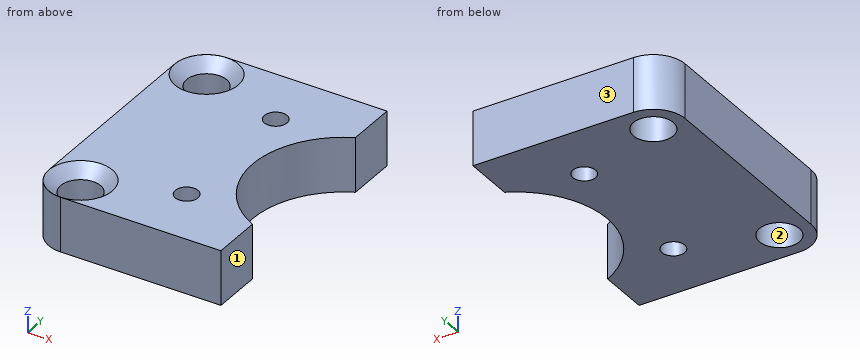
from build123d import *

# Parameters (mm, degrees)
SKETCH_R     = 2.2
SKETCH_R_2   = 1.25
PAD_DEPTH    = 6
CHAMFER_SIZE = 1.29


with BuildPart() as part:
    # Sketch → Pad (new body)
    with BuildSketch(Plane.XY):
        with BuildLine():
            Line((0, 14.5), (17.63, 14.5))
            Line((17.63, 14.5), (17.63, 8.994615))
            ThreePointArc((17.63, 8.994615), (12, 0), (17.63, -8.994615))
            Line((17.63, -8.994615), (17.63, -14.5))
            Line((17.63, -14.5), (0, -14.5))
            ThreePointArc((-3.5, -11), (-2.474874, -13.474874), (0, -14.5))
            Line((-3.5, -11), (-3.5, 11))
            ThreePointArc((0, 14.5), (-2.474874, 13.474874), (-3.5, 11))
        make_face()
        with Locations((0, 11)):
            Circle(SKETCH_R, mode=Mode.SUBTRACT)
        with Locations((0, -11)):
            Circle(SKETCH_R, mode=Mode.SUBTRACT)
        with Locations((9.63, 7.78)):
            Circle(SKETCH_R_2, mode=Mode.SUBTRACT)
        with Locations((9.63, -7.78)):
            Circle(SKETCH_R_2, mode=Mode.SUBTRACT)
    extrude(amount=PAD_DEPTH)

    # Chamfer
    chamfer_edges = [part.edges().sort_by_distance(p)[0] for p in [
        (-2.2, -11, 6),
        (-2.2, 11, 6),
    ]]
    chamfer(chamfer_edges, length=CHAMFER_SIZE)


solid = part.part
Work out the finished part from the listing and answer in its coordinate system (mm). Face numbers are marked on the shaded views. Round coordinates to 2 decimals unless told otherwise and drop trailing zeros. Write each loop counter-clockwise with the first axis right and the second up, starting at its lowest first coordinate (ties: lowest second). Pieces come first, ordered by that corner, then holes.
1) Given pin 1 Ø5 at (x, y) = (0, -11) entering from +Z; pin 2 Ø1 at (y, z) = (-2, 2) entering from +X; pin 3 Ø3 at (x, y) = (9.63, -7.78) entering from +Z, each flat-ended and moving along its own axis, determine where each tip first touches the part or whether it passes through.
2) Straight lines are drawn through the part: line 1 (Y direction, x = 9.63, z = 4.45); line 2 (Y direction, x = 0, z = 1.8); line 3 (X direction, y = 8.5, z = 0.7). For each, find the intervals that lie inside material, in ascending order.
3) A cutting plane is placed at C-C (y = 7). Give the vertices of the cut face in (x, z).
4) A cutting plane is placed at D-D (x = 13). Give the vertices of the cut face in (y, z).
5) A cutting plane is placed at B-B (z = 1.85). Give the vertices of the cut face in (x, y).
6) A cutting plane is placed at A-A (x = 9.63). Give the vertices of the cut face in (y, z), plus the area to 3 significant figures.
7) The mould has two halves that part along Y. Classify the marked faces 1, 2 and 3: pulls with the +Y half, pulls with the -Y half, needs draft (parallel to the pull), parting line crosses it, or undercut.
Completed:
1. pin 1: stops at z = 5.01
1. pin 2: stops at x = 12.32
1. pin 3: stops at z = 6
2. line 1: y = -14.5 to -9.03, -6.53 to 6.53, 9.03 to 14.5
2. line 2: y = -14.5 to -13.2, -8.8 to 8.8, 13.2 to 14.5
2. line 3: x = -3.5 to 8.61, 10.65 to 16.73
3. outline: (-3.5, 0) - (8.65, 0) - (8.65, 6) - (-3.5, 6) - close; (10.61, 0) - (14.86, 0) - (14.86, 6) - (10.61, 6) - close
4. outline: (-14.5, 0) - (-4.36, 0) - (-4.36, 6) - (-14.5, 6) - close; (4.36, 0) - (14.5, 0) - (14.5, 6) - (4.36, 6) - close
5. outline: (-3.5, -11) arc R3.5 ccw to (0, -14.5) - (17.63, -14.5) - (17.63, -8.99) arc R10 cw to (17.63, 8.99) - (17.63, 14.5) - (0, 14.5) arc R3.5 ccw to (-3.5, 11) - close; hole circle Ø4.4 at (0, -11); hole circle Ø4.4 at (0, 11); hole circle Ø2.5 at (9.63, -7.78); hole circle Ø2.5 at (9.63, 7.78)
6. outline: (-14.5, 0) - (-9.03, 0) - (-9.03, 6) - (-14.5, 6) - close; (-6.53, 0) - (6.53, 0) - (6.53, 6) - (-6.53, 6) - close; (9.03, 0) - (14.5, 0) - (14.5, 6) - (9.03, 6) - close
6. area: 144 mm2
7. face 1: needs draft
7. face 2: undercut
7. face 3: pulls with the +Y half
